The listing builds one solid part. Answer for the finished solid, in the listing's coordinates (mm). Face numbers are marked on the shaded views. Round coordinates to 2 decimals unless told otherwise and drop trailing zeros. Order: outer loops, then holes, each group sorted by start corner. A loop starts at its lowest first (then second) coordinate and runs counter-clockwise, first axis right, second up. Notation, with made-up numbers: (86.5, 19) - (137.5, 19) arc R22 cw to (137.5, 39) - close; hole circle Ø9 at (88, 9.5). An arc over 180 degrees is marked (long way). Use CSV: the item, a comma, the result in double quotes. Start each with the question number.
Item 1: Find section D-D, the plane y = 17.5. Give the vertices of the cut face in (x, z).
Item 2: Flat-ended cylindrical pins translate along their axes: P1, Ø5, axis at x = -36, z = 5, coming from the -Y side; P2, Ø3, axis at y = 23.5, z = 17.5, coming from the +X side; P3, Ø2, axis at x = -17.5, y = 6.5, coming from the -Z side; P4, Ø4, axis at y = 18, z = 9.5, coming from the -X side. Find the tip coordinate at first contact, or state that the pin passes through.
Item 3: Determine the mould class of the marked faces 1, 2 and 3 for opening direction X: +X half, -X half, draft (parallel to the pull), parting line (faces both ways), or undercut.
Item 4: Find section C-C, the plane z = 11. Count the separate pieces of the cut face and the enclosed holes in it, plus the area to 3 significant figures.
Item 5: Find section B-B, the plane y = 0. Give the vertices of the cut face in (x, z), plus the area to 3 significant figures.
Item 6: Find section A-A, the plane x = 0. Give the vertices of the cut face in (y, z).
Item 7: Straight lines are drawn through the part: line 1 along X through (y, z) = (-3, 15.75); line 2 along Y through (x, z) = (17.5, 23.5); line 3 along Y through (x, z) = (5.5, 9.5). For each, find the intervals that lie inside material, in ascending order. Write a range as [from, to].
```python
from build123d import *

# Parameters (mm, degrees)
SKETCH1_R           = 50
SKETCH1_R_2         = 12.5
BOSS_EXTRUDE1_DEPTH = 25


with BuildPart() as part:
    # Sketch1 → Boss-Extrude1 (new body)
    with BuildSketch(Plane.XY):
        Circle(SKETCH1_R)
        Circle(SKETCH1_R_2, mode=Mode.SUBTRACT)
        with BuildLine():
            Line((7.8897322, 21.071357949), (12.430935999, 38.019361254))
            ThreePointArc((12.430935999, 38.019361254), (0, 40), (-12.430935999, 38.019361254))
            Line((-12.430935999, 38.019361254), (-7.8897322, 21.071357949))
            ThreePointArc((-7.8897322, 21.071357949), (0, 22.5), (7.8897322, 21.071357949))
        make_face(mode=Mode.SUBTRACT)
        with BuildLine():
            Line((21.393418589, 6.96933577), (37.475295395, 13.985786895))
            ThreePointArc((37.475295395, 13.985786895), (31.273259299, 24.939592074), (21.974171749, 33.423581136))
            Line((21.974171749, 33.423581136), (11.555083457, 19.306217815))
            ThreePointArc((11.555083457, 19.306217815), (17.591208356, 14.028520542), (21.393418589, 6.96933577))
        make_face(mode=Mode.SUBTRACT)
        with BuildLine():
            Line((18.787424434, -12.380738392), (34.299993002, -20.579370255))
            ThreePointArc((34.299993002, -20.579370255), (38.997116487, -8.900837358), (39.832279979, 3.659162705))
            Line((39.832279979, 3.659162705), (22.29868559, 3.003101891))
            ThreePointArc((22.29868559, 3.003101891), (21.935878024, -5.006721014), (18.787424434, -12.380738392))
        make_face(mode=Mode.SUBTRACT)
        with BuildLine():
            Line((2.034116487, -22.407864024), (5.296096286, -39.64784186))
            ThreePointArc((5.296096286, -39.64784186), (17.355349565, -36.038754716), (27.695868954, -28.860679876))
            Line((27.695868954, -28.860679876), (16.250922663, -15.561411009))
            ThreePointArc((16.250922663, -15.561411009), (9.76238413, -20.271799528), (2.034116487, -22.407864024))
        make_face(mode=Mode.SUBTRACT)
        with BuildLine():
            Line((-16.250922663, -15.561411009), (-27.695868954, -28.860679876))
            ThreePointArc((-27.695868954, -28.860679876), (-17.355349565, -36.038754716), (-5.296096286, -39.64784186))
            Line((-5.296096286, -39.64784186), (-2.034116487, -22.407864024))
            ThreePointArc((-2.034116487, -22.407864024), (-9.76238413, -20.271799528), (-16.250922663, -15.561411009))
        make_face(mode=Mode.SUBTRACT)
        with BuildLine():
            Line((-22.29868559, 3.003101891), (-39.832279979, 3.659162705))
            ThreePointArc((-39.832279979, 3.659162705), (-38.997116487, -8.900837358), (-34.299993002, -20.579370255))
            Line((-34.299993002, -20.579370255), (-18.787424434, -12.380738392))
            ThreePointArc((-18.787424434, -12.380738392), (-21.935878024, -5.006721014), (-22.29868559, 3.003101891))
        make_face(mode=Mode.SUBTRACT)
        with BuildLine():
            Line((-11.555083457, 19.306217815), (-21.974171749, 33.423581136))
            ThreePointArc((-21.974171749, 33.423581136), (-31.273259299, 24.939592074), (-37.475295395, 13.985786895))
            Line((-37.475295395, 13.985786895), (-21.393418589, 6.96933577))
            ThreePointArc((-21.393418589, 6.96933577), (-17.591208356, 14.028520542), (-11.555083457, 19.306217815))
        make_face(mode=Mode.SUBTRACT)
    extrude(amount=BOSS_EXTRUDE1_DEPTH)


solid = part.part
```
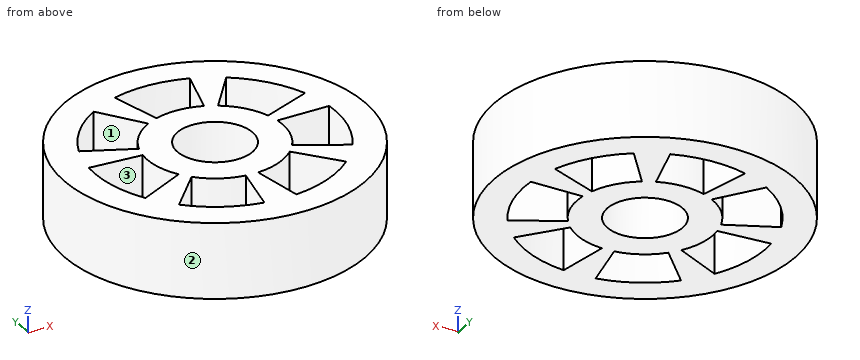
Worked out:
1,outline,"(-46.84, 0) - (-35.97, 0) - (-35.97, 25) - (-46.84, 25) - close; (-14.14, 0) - (14.14, 0) - (14.14, 25) - (-14.14, 25) - close; (35.97, 0) - (46.84, 0) - (46.84, 25) - (35.97, 25) - close"
2,P1,"stops at y = -37.12"
2,P2,"stops at x = 44.9"
2,P3,"stops at z = 0"
2,P4,"stops at x = -47.37"
3,face 1,"undercut"
3,face 2,"parting line"
3,face 3,"undercut"
4,separate pieces,"1"
4,enclosed holes,"8"
4,area,"4,830 mm²"
5,outline,"(-50, 0) - (-40, 0) - (-40, 25) - (-50, 25) - close; (-22.5, 0) - (-12.5, 0) - (-12.5, 25) - (-22.5, 25) - close; (12.5, 0) - (22.5, 0) - (22.5, 25) - (12.5, 25) - close; (40, 0) - (50, 0) - (50, 25) - (40, 25) - close"
5,area,"1,000 mm²"
6,outline,"(-50, 0) - (-12.5, 0) - (-12.5, 25) - (-50, 25) - close; (12.5, 0) - (22.5, 0) - (22.5, 25) - (12.5, 25) - close; (40, 0) - (50, 0) - (50, 25) - (40, 25) - close"
7,line 1,"x = [-49.91, -39.89], [-22.3, -12.13], [12.13, 22.3], [39.89, 49.91]"
7,line 2,"y = [-46.84, -35.97], [-17.01, 14.14], [27.36, 46.84]"
7,line 3,"y = [-49.7, -39.62], [-21.82, -11.22], [11.22, 21.82], [39.62, 49.7]"
